from build123d import *

# Parameters (mm, degrees)
F1_DEPTH = 152.4


with BuildPart() as f1:
    # F0 (on Front) → F1 (new body)
    with BuildSketch(Plane.XZ):
        with BuildLine():
            Line((-50.8, -73.025), (-25.4, -73.025))
            Line((-25.4, -73.025), (-25.4, -69.240349))
            Line((-25.4, -69.240349), (-50.8, -69.240349))
            ThreePointArc((-50.8, -69.240349), (-120.040349, 0), (-50.8, 69.240349))
            Line((-50.8, 69.240349), (-25.4, 69.240349))
            Line((-25.4, 69.240349), (-25.4, 73.025))
            Line((-25.4, 73.025), (-50.8, 73.025))
            ThreePointArc((-50.8, 73.025), (-123.825, 0), (-50.8, -73.025))
        make_face()
        with BuildLine():
            Line((-25.4, -73.025), (0, -73.025))
            ThreePointArc((0, -73.025), (73.025, 0), (0, 73.025))
            Line((0, 73.025), (-25.4, 73.025))
            Line((-25.4, 73.025), (-25.4, 69.240349))
            Line((-25.4, 69.240349), (0, 69.240349))
            ThreePointArc((0, 69.240349), (69.240349, 0), (0, -69.240349))
            Line((0, -69.240349), (-25.4, -69.240349))
            Line((-25.4, -69.240349), (-25.4, -73.025))
        make_face()
    extrude(amount=F1_DEPTH)


solid = f1.part
Build history of the part. All positions in model axes, mm. A direction names the side the tool comes from. Coordinates: 2 decimals unless noted, no trailing zeros. Order: outer loops, then holes, each group sorted by start corner. A loop starts at its lowest first (then second) coordinate and runs counter-clockwise, first axis right, second up. Notation, with made-up numbers: M 46.25,-34 L 56.25,-34 A6 cw 56.25,-29 Z; hole C 83,-35.5 d10. An arc over 180 degrees is marked long. One line per question, with ' | ' between items. Start each with the question number.
Q1. Saw through at A-A (z = 0). List the corners of the cut face in (x, y) (3 decimals).
Q2. Saw through at C-C (y = -35.5). List the corners of the cut face in (x, z) (3 decimals), then the cut area to 3 significant figures.
Q3. Probe L1, parallel to Z at x = -37.5, y = -39.5 (3 decimals); L2, parallel to X at y = -56, z = 28; L3, parallel to Z at x = 33, y = -80.5. List the from-to ranges inside material, lowest first. Write a range as from..to.
Q4. 3-axis set-ups, long thin cutter, end or side, ignore diameter. For faces 1 (the face through (-26, -75, 69.24)), 2 (the face through (-26, -75, -73.025)): which of +Z, -Z, +X, -X, +Y, -Y reach the whole face in a straight line?
Q5. Saw through at B-B (x = -3.5). List the corners of the cut face in (y, z) (3 decimals), then the cut area to 3 significant figures.
Q6. Flat gauge pins, fed straight in: pin 1 Ø2 at (y, z) = (-76.5, 25.5) entering from -X; pin 2 Ø5 at (x, y) = (-97.5, -37) entering from -Z; pin 3 Ø4 at (y, z) = (-62, 48.5) entering from -X. Where does each tip first touch, or does it go through?
Q7. Two-plate mould, pull along X, no slides. Class faces 3 (the face through (-26, 0, -70)), 4 (the face through (-25, -75, -69.24)), 5 (the face through (69.224, -75.133, 1.523)), 6 (the face through (-123.807, -75.133, 1.606)): +X half, -X half, draft (parallel to the pull), parting line (faces both ways), or undercut.
Check values:
1) outline: M -123.825,-152.4 L -120.04,-152.4 L -120.04,0 L -123.825,0 Z; M 69.24,-152.4 L 73.025,-152.4 L 73.025,0 L 69.24,0 Z
2) outline: M -50.8,-73.025 L 0,-73.025 A73.025 ccw 0,73.025 L -50.8,73.025 A73.025 ccw Z; hole M -50.8,-69.24 L 0,-69.24 A69.24 ccw 0,69.24 L -50.8,69.24 A69.24 ccw Z | area: 2,080 mm2
3) L1: z = -73.025..-69.24, 69.24..73.025 | L2: x = -118.24..-114.13, 63.33..67.44 | L3: z = -65.14..-60.87, 60.87..65.14
4) face 1: +Y, -Y | face 2: -Z, +X, -X, +Y, -Y
5) outline: M -152.4,-73.025 L 0,-73.025 L 0,-69.24 L -152.4,-69.24 Z; M -152.4,69.24 L 0,69.24 L 0,73.025 L -152.4,73.025 Z | area: 1,150 mm2
6) pin 1: stops at x = -119.59 | pin 2: stops at z = -58.13 | pin 3: stops at x = -107.11
7) face 3: draft | face 4: undercut | face 5: undercut | face 6: -X half
